Check sheet for the modelled part. Datum: model origin and axes. Units: mm. A direction names the side the tool comes from. Give positions to 0.01 mm unless a question says otherwise; leave off trailing zeros. Write each loop counter-clockwise with the first axis right and the second up, starting at its lowest first coordinate (ties: lowest second). Pieces come first, ordered by that corner, then holes.
from build123d import *


with BuildPart() as part:
    # Sketch1 → Revolve2 (revolve)
    with BuildSketch(Plane(origin=(0, 0, 0), x_dir=(0, 0, -1), z_dir=(1, 0, 0)), mode=Mode.PRIVATE) as revolve2_sk:
        with BuildLine():
            Line((310.023918284, 20), (310.023918284, 0))
            Line((310.023918284, 0), (320.023918284, 0))
            Line((320.023918284, 0), (320.023918284, 20))
            ThreePointArc((320.023918284, 20), (317.094986096, 27.071067812), (310.023918284, 30))
            Line((310.023918284, 30), (290.064881334, 30))
            ThreePointArc((290.064881334, 30), (279.487694994, 30.939665349), (269.24180917, 33.729229029))
            Line((269.24180917, 33.729229029), (149.24180917, 78.135385485))
            ThreePointArc((149.24180917, 78.135385485), (144.118866258, 79.530167326), (138.830273088, 80))
            Line((138.830273088, 80), (-161.169726912, 80))
            ThreePointArc((-161.169726912, 80), (-167.788864689, 77.49579983), (-171.092873277, 71.237403019))
            Line((-171.092873277, 71.237403019), (-179.976081716, 0))
            Line((-179.976081716, 0), (-169.898632858, 0))
            Line((-169.898632858, 0), (-161.169726912, 70))
            Line((-161.169726912, 70), (138.830273088, 70))
            ThreePointArc((138.830273088, 70), (142.356001868, 69.686778217), (145.771297142, 68.756923657))
            Line((145.771297142, 68.756923657), (265.771297142, 24.350767201))
            ThreePointArc((265.771297142, 24.350767201), (277.724830603, 21.09627624), (290.064881334, 20))
            Line((290.064881334, 20), (310.023918284, 20))
        make_face()
    revolve(revolve2_sk.sketch.rotate(Axis((0, 0, 179.976081716), (0, 0, -1)), 180), axis=Axis((0, 0, 179.976081716), (0, 0, -1)))


solid = part.part
1) Gauge pin test, flat ends, axial feed: pin 1 (6 mm diameter, centred on x = -40.5, z = -117.5, fed in from +Y); pin 2 (6 mm diameter, centred on y = -39, z = -63.5, fed in from +X); pin 3 (1 mm diameter, centred on y = -40.5, z = 113.5, fed in from +X). Record the tip position at first contact, or that the pin passes through.
2) Scan lines: L1, parallel to X at y = 0, z = -76; L2, parallel to Y at x = 26.5, z = -13.5; L3, parallel to Z at x = 2, y = 4. Record each from-to range of solid material in increasing order.
3) Sectioned sample at A-A on z = 132. Record the boundary of the cut face in (x, y), then the cut area to 3 significant figures.
4) Sectioned sample at B-B on z = -173.5. Record the boundary of the cut face in (x, y), then the cut area to 3 significant figures.
5) Draft check along X on faces 4 (the conical face through (3.377, 0.75, 179.545)), 5 (the flat face through (0, 0, -320.024)), 6 (the cylindrical face through (-0.88, 19.98, -300.18)). Enter one of: +X half, -X half, draft (parallel to the pull), parting line (faces both ways), or undercut.
6) Access from +Z, -Z, +X, -X, +Y, -Y to the whole of each face (thin tool, end or side, straight path). Record for faces 1 (the cylindrical face through (-3.517, 79.923, 13.27)), 2 (the cylindrical face through (-25.296, -16.128, -299.905)), 3 (the cylindrical face through (68.335, 15.175, 9.07)).
Answers below:
1. pin 1: stops at y = 70.67
1. pin 2: stops at x = 71.44
1. pin 3: stops at x = 69.28
2. L1: x = -80 to -70, 70 to 80
2. L2: y = -75.48 to -64.79, 64.79 to 75.48
2. L3: z = -320.02 to -310.02, 169.34 to 179.42
3. outline: circle Ø160 at (0, 0); hole circle Ø140 at (0, 0)
3. area: 4,710 mm2
4. outline: circle Ø138.32 at (0, 0); hole circle Ø116.99 at (0, 0)
4. area: 4,280 mm2
5. face 4: parting line
5. face 5: draft
5. face 6: undercut
6. face 1: +Z, -Z
6. face 2: -Z
6. face 3: none
